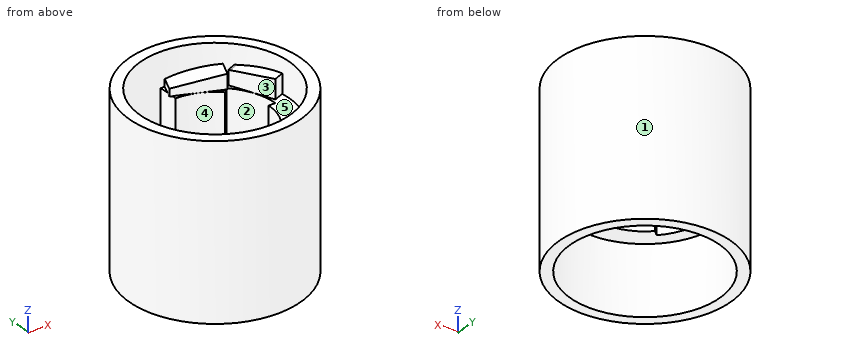
from build123d import *

# Parameters (mm, degrees)
SKETCH1_R                = 25
SKETCH1_R_2              = 21.775
BOSS_EXTRUDE1_DEPTH      = 50
BOSS_EXTRUDE2_START      = -20
BOSS_EXTRUDE2_DEPTH      = 20
BOSS_EXTRUDE3_REACH      = 60.561
BOSS_EXTRUDE4_REACH      = 62.226
BOSS_EXTRUDE4_END_RADIUS = 21.775


with BuildPart() as part:
    # Sketch1 → Boss-Extrude1 (new body)
    with BuildSketch(Plane.XY):
        Circle(SKETCH1_R)
        Circle(SKETCH1_R_2, mode=Mode.SUBTRACT)
    extrude(amount=BOSS_EXTRUDE1_DEPTH)

    # Sketch2 → Boss-Extrude2 (add)
    with BuildSketch(Plane(origin=(0, 0, 0), x_dir=(-1, 0, 0), z_dir=(0, 0, -1)).offset(BOSS_EXTRUDE2_START)):
        with BuildLine():
            Line((0, -15.77607933), (0, -21.775))
            ThreePointArc((0, -21.775), (8.33293174, -20.11747682), (15.39725016, -15.39725016))
            Line((15.39725016, -15.39725016), (12.569586237, -12.569586237))
            Line((12.569586237, -12.569586237), (11.198401724, -11.198401724))
            Line((11.198401724, -11.198401724), (11.155372675, -11.155372675))
            ThreePointArc((11.155372675, -11.155372675), (6.037244187, -14.575196796), (0, -15.77607933))
        make_face()
        with BuildLine():
            Line((12.569586237, -12.569586237), (15.39725016, -15.39725016))
            ThreePointArc((15.39725016, -15.39725016), (20.11747682, -8.33293174), (21.775, 0))
            Line((21.775, 0), (17.77607933, 0))
            ThreePointArc((17.77607933, 0), (16.422955861, -6.802611052), (12.569586237, -12.569586237))
        make_face()
        with BuildLine():
            ThreePointArc((21.775, 0), (20.11747682, 8.33293174), (15.39725016, 15.39725016))
            Line((15.39725016, 15.39725016), (11.155372675, 11.155372675))
            ThreePointArc((11.155372675, 11.155372675), (14.575196796, 6.037244187), (15.77607933, 0))
            Line((15.77607933, 0), (17.77607933, 0))
            Line((17.77607933, 0), (21.775, 0))
        make_face()
        with BuildLine():
            ThreePointArc((0, 21.775), (-8.33293174, 20.11747682), (-15.39725016, 15.39725016))
            Line((-15.39725016, 15.39725016), (-12.568823036, 12.568823036))
            Line((-12.568823036, 12.568823036), (-11.154609473, 11.154609473))
            ThreePointArc((-11.154609473, 11.154609473), (-6.036831146, 14.574199625), (0, 15.775))
            Line((0, 15.775), (0, 21.775))
        make_face()
        with BuildLine():
            ThreePointArc((-15.39725016, 15.39725016), (-20.11747682, 8.33293174), (-21.775, 0))
            Line((-21.775, 0), (-17.775, 0))
            ThreePointArc((-17.775, 0), (-16.42195869, 6.80219801), (-12.568823036, 12.568823036))
            Line((-12.568823036, 12.568823036), (-15.39725016, 15.39725016))
        make_face()
        with BuildLine():
            Line((-17.775, 0), (-21.775, 0))
            ThreePointArc((-21.775, 0), (-20.11747682, -8.33293174), (-15.39725016, -15.39725016))
            Line((-15.39725016, -15.39725016), (-11.154609473, -11.154609473))
            ThreePointArc((-11.154609473, -11.154609473), (-14.574199625, -6.036831146), (-15.775, 0))
            Line((-15.775, 0), (-17.775, 0))
        make_face()
    extrude(amount=-BOSS_EXTRUDE2_DEPTH)

    # Sketch3 → Boss-Extrude3 (add, up to next)
    with BuildSketch(Plane(origin=(6.036831146, 14.574199625, 20), x_dir=(-0.9238795325112862, 0.38268343236509134, 0), z_dir=(-0.38268343236509134, -0.9238795325112862, 0)), mode=Mode.PRIVATE) as boss_extrude3_sk1:
        Polygon((7.280816653, -19.963261278), (-6.92881971, -19.963261278), (-6.92881971, -24.309436753), (7.280816653, -22.136349016), align=None)
    boss_extrude3_tool1 = extrude(boss_extrude3_sk1.sketch, amount=-BOSS_EXTRUDE3_REACH, mode=Mode.PRIVATE) - part.part
    add(boss_extrude3_tool1.solids().sort_by_distance((6.603563, 14.339452, 41.653441))[0])

    # Boss-Extrude4: up to this cylinder (the profile starts inside it)
    boss_extrude4_end = Plane(origin=(0, 0, 42.508231), z_dir=(0, 0, -1)) * Cylinder(BOSS_EXTRUDE4_END_RADIUS, 169.002, mode=Mode.PRIVATE)
    # Sketch4 → Boss-Extrude4 (add, up to the surface)
    with BuildSketch(Plane(origin=(16.42195869, 6.80219801, 20), x_dir=(0, 0, 1), z_dir=(-0.9238795325112876, -0.38268343236508784, 0)), mode=Mode.PRIVATE) as boss_extrude4_sk1:
        Polygon((24.315182013, 6.595374184), (25.634239275, -5.93507645), (20.034984376, -5.93507645), (20.034984376, 7.085544356), (24.315182013, 7.085544356), align=None)
    boss_extrude4_tool1 = extrude(boss_extrude4_sk1.sketch, amount=-BOSS_EXTRUDE4_REACH, mode=Mode.PRIVATE) & boss_extrude4_end
    add(boss_extrude4_tool1.solids().sort_by_distance((16.317145, 7.05524, 42.508231))[0])


solid = part.part
Check sheet for the modelled part. Datum: model origin and axes. Units: mm. Face numbers are marked on the shaded views. A direction names the side the tool comes from. Round coordinates to 2 decimals unless told otherwise and drop trailing zeros. Order: outer loops, then holes, each group sorted by start corner. A loop starts at its lowest first (then second) coordinate and runs counter-clockwise, first axis right, second up.
(1) Go/stop test with flat-tipped pins: P1, Ø3, axis at x = 3.5, y = 16, coming from the +Z side; P2, Ø0.5, axis at x = 16, y = 13.5, coming from the +Z side; P3, Ø1.7, axis at x = 9, y = 13.5, coming from the +Z side. Record where each tip stops, or that it passes through.
(2) Access from +Z, -Z, +X, -X, +Y, -Y to the whole of each face (thin tool, end or side, straight path). Record for the marked faces 3, 4 and 5.
(3) Scan lines: probe 1 along Y at (x, z) = (0, 10) (3 decimals); probe 2 along Z at (x, y) = (-19, 4); probe 3 along Y at (x, z) = (14, 27). Record each from-to range of solid material in increasing order.
(4) Cross-section at B-B, the plane y = -6.5. Enter the section's corners in (x, z), and give its area (3 significant figures).
(5) Cross-section at C-C, the plane z = 15. Enter the section's corners in (x, y) (3 decimals), and give its area (3 significant figures).
(6) Draft check along X on the marked faces 1 and 2. Enter one of: pulls with the +X half, pulls with the -X half, needs draft (parallel to the pull), parting line crosses it, or undercut.
(7) Cross-section at A-A, the plane z = 33.5. Enter the section's corners in (x, y) (3 decimals).
Check sheet entries:
1. P1: stops at z = 43.04
1. P2: stops at z = 44.37
1. P3: stops at z = 43.86
2. face 3: +Z
2. face 4: +Z, -Z
2. face 5: none
3. probe 1: y = -25 to -21.775, 21.775 to 25
3. probe 2: z = 20 to 40
3. probe 3: y = -20.71 to -16.68, -14 to -7.27, 10.95 to 20.71
4. outline: (-24.14, 0) - (-20.78, 0) - (-20.78, 20) - (-16.55, 20) - (-16.55, 40) - (-20.78, 40) - (-20.78, 50) - (-24.14, 50) - close; (14.37, 20) - (20.78, 20) - (20.78, 0) - (24.14, 0) - (24.14, 50) - (20.78, 50) - (20.78, 40) - (14.37, 40) - close
4. area: 549 mm2
5. outline: circle Ø50 at (0, 0); hole circle Ø43.55 at (0, 0)
5. area: 474 mm2
6. face 1: parting line crosses it
6. face 2: undercut
7. outline: circle Ø50 at (0, 0); hole (-17.776, 0) arc R17.776 ccw to (-12.57, -12.57) - (-11.155, -11.155) arc R15.776 ccw to (0, -15.776) - (0, -21.775) arc R21.775 ccw to (15.397, -15.397) - (11.155, -11.155) arc R15.775 ccw to (15.775, 0) - (17.775, 0) arc R17.775 ccw to (12.569, 12.569) - (11.155, 11.155) arc R15.775 ccw to (0, 15.775) - (0, 21.775) arc R21.775 ccw to (-15.397, 15.397) - (-11.155, 11.155) arc R15.776 ccw to (-15.776, 0) - close
